from build123d import *

# Parameters (mm, degrees)
F0_R            = 15.8688012495
F0_R_2          = 1.7272
F0_R_3          = 3.96875
F1_DEPTH        = 3.175
F3_DEPTH        = 3.175
F3_COPIES_COUNT = 32


# Not quite as in the source:
# - a pattern or mirror of a feature is missing from the dataset's text; its kind, count and spacing are read off the source's solid


with BuildPart() as f1:
    # F0 (on Top) → F1 (new body)
    with BuildSketch(Plane.XY):
        Circle(F0_R)
        with Locations((0, -9.525)):
            Circle(F0_R_2, mode=Mode.SUBTRACT)
        Circle(F0_R_3, mode=Mode.SUBTRACT)
        with Locations((0, 9.525)):
            Circle(F0_R_2, mode=Mode.SUBTRACT)
    extrude(amount=F1_DEPTH)

    # F2 (on face) → F3 (cut, through all)
    with BuildSketch(Plane.XY.offset(3.175)):
        with BuildLine():
            Line((-13.9312413972, 0.274735453), (-15.8329891451, 1.065508248))
            ThreePointArc((-15.8329891451, 1.065508248), (-15.8688012495, 0), (-15.8329891451, -1.065508248))
            Line((-15.8329891451, -1.065508248), (-13.9312413972, -0.274735453))
            ThreePointArc((-13.9312413972, -0.274735453), (-13.747940143, 0), (-13.9312413972, 0.274735453))
        make_face()
    f3 = extrude(amount=-F3_DEPTH, mode=Mode.SUBTRACT)

    # F3_copies: F3 ×32 about axis
    f3_copies_axis = Axis((0, 0, 0), (0, 0, 1))
    for i in range(1, F3_COPIES_COUNT):
        add(f3.rotate(f3_copies_axis, i * 360 / F3_COPIES_COUNT), mode=Mode.SUBTRACT)


solid = f1.part
Verification items for the finished model (mm, model axes). A direction names the side the tool comes from. Give positions to 0.01 mm unless a question says otherwise; leave off trailing zeros. Loops run counter-clockwise (first coordinate to the right, second up) from the corner with the lowest first, then second, coordinate; pieces in that order, holes last.
1) Depth check by flat-ended pin: pin 1 Ø1.5 at (x, z) = (5.5, 0.5) entering from -Y; pin 2 Ø8 at (x, y) = (10.5, 3.5) entering from -Z; pin 3 Ø1.5 at (x, z) = (5, 2.5) entering from +Y; pin 4 Ø1 at (x, z) = (-3, 1.5) entering from +Y (3 decimals). Enter the tip coordinate at first touch or a pass-through.
2) Sectioned sample at B-B, the plane x = 3.5. Enter the section's corners in (y, z) (3 decimals), then the cut area to 3 significant figures.
3) Sectioned sample at C-C, the plane z = 1.55. Count the separate pieces of the cut face and the enclosed holes in it, then the cut area to 3 significant figures.
4) Sectioned sample at A-A, the plane y = 1.5. Enter the section's corners in (x, z) (3 decimals), then the cut area to 3 significant figures.
5) Thickness scan on line 1 along Y through (x, z) = (0, 2.2); line 2 along X through (y, z) = (12, 0.8); line 3 along X through (y, z) = (-13, 0.75). Record the ranges inside material, lowest first.
6) Draft check along Y on faces 6 (the cylindrical face through (7.49, 13.99, 1.57)), 7 (the flat face through (14.45, -3.55, 1.61)), 8 (the cylindrical face through (7.47, -14, 1.57)). Enter one of: pulls with the +Y half, pulls with the -Y half, needs draft (parallel to the pull), parting line crosses it, or undercut.
7) Set-up check for faces 1 (the flat face through (-6.3, -13.48, 1.61)), 2 (the flat face through (-13.48, 6.3, 1.61)), 3 (the flat face through (7.7, -12.7, 1.6)), 4 (the flat face through (-6.32, 13.5, 1.61)), 5 (the flat face through (14.48, 3.57, 1.61)): record each of +Z, -Z, +X, -X, +Y, -Y from which the full face is reachable in a straight line by a thin tool's end or side.
Answers:
1. pin 1: stops at y = -15.14
1. pin 2: stops at z = 0
1. pin 3: stops at y = 15.29
1. pin 4: stops at y = 14.375
2. outline: (-14.375, 0) - (-1.871, 0) - (-1.871, 3.175) - (-14.375, 3.175) - close; (1.871, 0) - (14.375, 0) - (14.375, 3.175) - (1.871, 3.175) - close
2. area: 79.4 mm2
3. separate pieces: 1
3. enclosed holes: 3
3. area: 637 mm2
4. outline: (-15.798, 0) - (-3.674, 0) - (-3.674, 3.175) - (-15.798, 3.175) - close; (3.674, 0) - (15.798, 0) - (15.798, 3.175) - (3.674, 3.175) - close
4. area: 77.0 mm2
5. line 1: y = -13.75 to -11.25, -7.8 to -3.97, 3.97 to 7.8, 11.25 to 13.75
5. line 2: x = -10.38 to -8.82, -7.56 to 7.56, 8.82 to 10.38
5. line 3: x = -7.76 to -5.82, -5.08 to 5.08, 5.82 to 7.76
6. face 6: pulls with the +Y half
6. face 7: undercut
6. face 8: pulls with the -Y half
7. face 1: +Z, -Z, -Y
7. face 2: +Z, -Z, -X
7. face 3: +Z, -Z
7. face 4: +Z, -Z, +Y
7. face 5: +Z, -Z, +X
